Geometry: see drawing. Coordinates: mm, zero at the bounding-box minimum. A direction names the side the tool comes from. Give positions to 0.01 mm unless a question says otherwise; leave off trailing zeros. Write each loop counter-clockwise with the first axis right and the second up, starting at its lowest first coordinate (ties: lowest second). Pieces come first, ordered by that corner, then holes. Notation, with made-up numbers: (19, 39.25) - (41, 39.25) arc R18 ccw to (41, 59.25) - close; hole circle Ø11 at (3.5, 70). An arc over 180 degrees is marked (long way). Return JSON: item names as keys, results as strings.
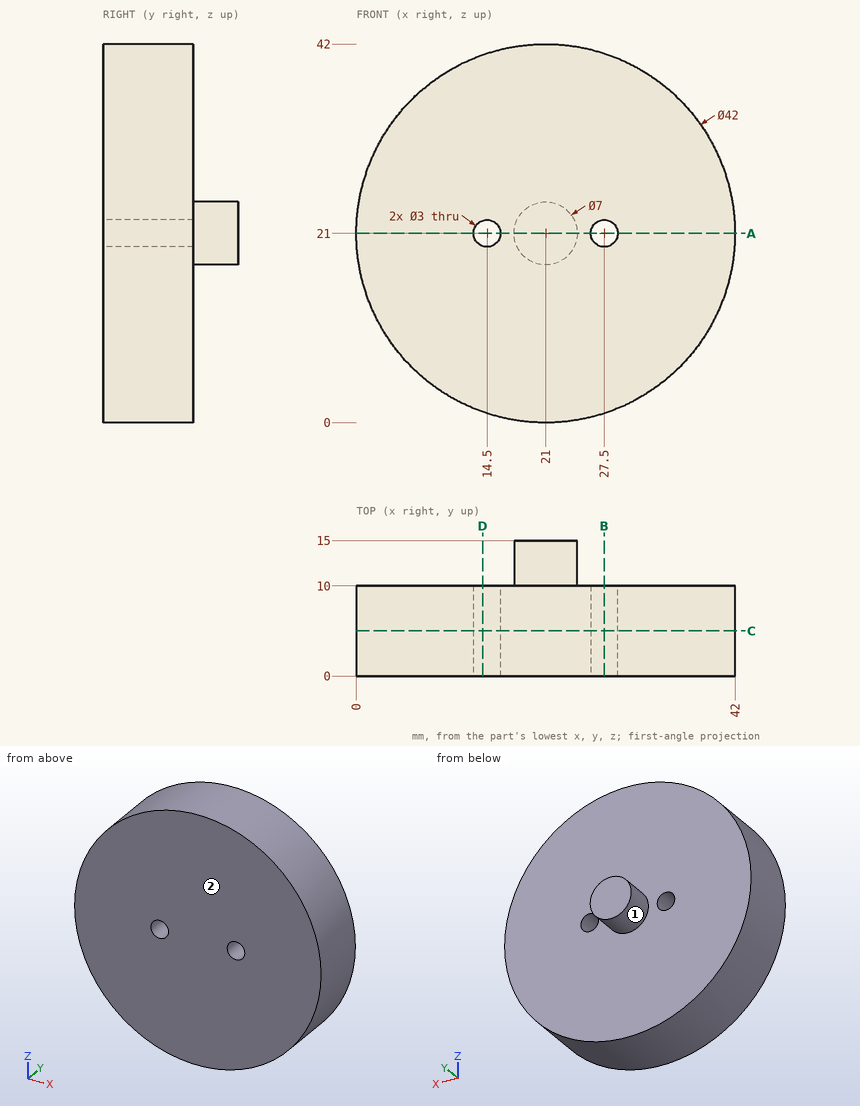
Q1. Section query B-B, the plane x = 27.5. Return the cut outline in (y, z).
Answer key:
{"outline": "(0, 1.03) - (10, 1.03) - (10, 19.5) - (0, 19.5) - close; (0, 22.5) - (10, 22.5) - (10, 40.97) - (0, 40.97) - close"}
Q2. Material intervals for probe 1 along X at (y, z) = (6.25, 21); probe 2 along Y at (x, z) = (22.5, 27); probe 3 along Z at (x, y) = (14.5, 3.75), sorted ascending. Write a range as [from, to].
Answer key:
{"probe 1": "x = [0, 13], [16, 26], [29, 42]", "probe 2": "y = [0, 10]", "probe 3": "z = [1.03, 19.5], [22.5, 40.97]"}
Q3. Section query A-A, the plane z = 21. Return the cut outline in (x, y), plus the area to 3 significant figures.
Answer key:
{"outline": "(0, 0) - (13, 0) - (13, 10) - (0, 10) - close; (16, 0) - (26, 0) - (26, 10) - (24.5, 10) - (24.5, 15) - (17.5, 15) - (17.5, 10) - (16, 10) - close; (29, 0) - (42, 0) - (42, 10) - (29, 10) - close", "area": "395 mm^2"}
Q4. Pin query (flat end, axial travel): P1, Ø5, axis at x = 27.5, z = 21, coming from the +Y side; P2, Ø2, axis at x = 8.5, y = 3, coming from the +Z side; P3, Ø1.5, axis at y = 6.5, z = 26, coming from the -X side. Return the tip coordinate at first contact, or that it passes through.
Answer key:
{"P1": "stops at y = 10", "P2": "stops at z = 38.57", "P3": "stops at x = 0.43"}
Q5. Section query D-D, the plane x = 14. Return the cut outline in (y, z), plus the area to 3 significant figures.
Answer key:
{"outline": "(0, 1.2) - (10, 1.2) - (10, 19.59) - (0, 19.59) - close; (0, 22.41) - (10, 22.41) - (10, 40.8) - (0, 40.8) - close", "area": "368 mm^2"}
Q6. Section query C-C, the plane y = 5. Return the cut outline in (x, z), plus the area to 3 significant figures.
Answer key:
{"outline": "circle Ø42 at (21, 21); hole circle Ø3 at (14.5, 21); hole circle Ø3 at (27.5, 21)", "area": "1,370 mm^2"}
Q7. Set-up query: the marked faces 1 and 2. Return all of +Z, -Z, +X, -X, +Y, -Y with unobstructed straight access to the full face (end or side cutting, diameter ignored); none if empty.
Answer key:
{"face 1": "+Y", "face 2": "+Z, -Z, +X, -X, -Y"}
